```python
from build123d import *


with BuildPart() as part:
    # Sketch1 → Revolve1 (revolve)
    with BuildSketch(Plane.XY):
        with BuildLine():
            Line((-90, 3), (-90, 1.77))
            Line((-90, 1.77), (-102.25, 1.77))
            Line((-102.25, 1.77), (-102.25, 1.16))
            Line((-102.25, 1.16), (-107.67, 1.16))
            Line((-107.67, 1.16), (-111.17, 0.5))
            ThreePointArc((-111.17, 0.5), (-111.523553391, 0.353553391), (-111.67, 0))
            Line((-111.67, 0), (0, 0))
            Line((0, 0), (0, 3))
            Line((0, 3), (-90, 3))
        make_face()
    revolve(axis=Axis((0, 0, 0), (-1, 0, 0)))


solid = part.part
```
Input: part model. Units: mm. Frame: model coordinates. A direction names the side the tool comes from. Give positions to 0.01 mm unless a question says otherwise; leave off trailing zeros. Order: outer loops, then holes, each group sorted by start corner. A loop starts at its lowest first (then second) coordinate and runs counter-clockwise, first axis right, second up. Notation, with made-up numbers: (17, -23) - (66, -23) arc R16 cw to (66, 8) - close; hole circle Ø2 at (67, 59). An arc over 180 degrees is marked (long way). Put each result on its own line as item: value.
Item 1: Section query A-A, the plane x = -12. Return loops of the section in (y, z).
Found:
outline: circle Ø6 at (0, 0)
Item 2: Access query for faces 1 (the flat face through (0, 0, 0)), 2 (the cylindrical face through (-96.21, 1.69, -0.53)). Directions: +Z, -Z, +X, -X, +Y, -Y. A direction counts if a zero-diameter tool reaches every point of the face in a straight line with its end or side. Return the directions, or none.
Found:
face 1: +Z, -Z, +X, +Y, -Y
face 2: -X
Item 3: Ray query, L1, parallel to X at y = -0.05, z = 2.15; L2, parallel to Y at x = -59.5, z = -0.3; L3, parallel to Z at x = -94.5, y = 0.1. Return the intervals inside material, ascending. Write a range as from..to.
Found:
L1: x = -90..0
L2: y = -2.98..2.98
L3: z = -1.77..1.77
Item 4: Contact query for flat-ended pins moving along their axis: pin 1 (2 mm diameter, centred on x = -72.5, z = 1.5, fed in from +Y); pin 2 (2 mm diameter, centred on x = -37, y = -1.5, fed in from -Z); pin 3 (3 mm diameter, centred on x = -88, y = 2.5, fed in from -Z). Output: stop coordinate, or through.
Found:
pin 1: stops at y = 2.96
pin 2: stops at z = -2.96
pin 3: stops at z = -2.83
